```python
from build123d import *

# Parameters (mm, degrees)
F0_R     = 1
F1_DEPTH = 6.5


with BuildPart() as f1:
    # F0 (on Front) → F1 (new body)
    with BuildSketch(Plane.XZ):
        with BuildLine():
            ThreePointArc((-35.216109, -69.5), (-37.643365, -66.55518), (-40.997419, -68.375582))
            ThreePointArc((-40.997419, -68.375582), (-39.352976, -72.276245), (-35.444986, -70.649293))
            ThreePointArc((-35.444986, -70.649293), (-35.273885, -70.085931), (-35.216109, -69.5))
        make_face()
        with BuildLine():
            Line((4, 9.5), (-4, 9.5))
            Line((-4, 9.5), (-4, -6.441955))
            ThreePointArc((-4, -6.441955), (-4.516669, -9.27034), (-5.999941, -11.73339))
            ThreePointArc((-5.999941, -11.73339), (-25.901345, -38.569953), (-40.997419, -68.375582))
            ThreePointArc((-40.997419, -68.375582), (-37.643365, -66.55518), (-35.216109, -69.5))
            ThreePointArc((-35.216109, -69.5), (-35.273885, -70.085931), (-35.444986, -70.649293))
            ThreePointArc((-35.444986, -70.649293), (-18.875971, -40.819152), (4, -15.5))
            Line((4, -15.5), (4, -9.5))
            Line((4, -9.5), (4, 9.5))
        make_face()
        with Locations((0, -12.5)):
            Circle(F0_R, mode=Mode.SUBTRACT)
    extrude(amount=F1_DEPTH)


solid = f1.part
```
Check sheet for the modelled part. Datum: model origin and axes. Units: mm. Round coordinates to 2 decimals unless told otherwise and drop trailing zeros. Order: outer loops, then holes, each group sorted by start corner. A loop starts at its lowest first (then second) coordinate and runs counter-clockwise, first axis right, second up.
1) Section check C-C (z = -12.5). Record the boundary of the cut face in (x, y).
2) Scan lines: line 1 (X direction, y = -4, z = -1); line 2 (Z direction, x = 0, y = -3); line 3 (Z direction, x = -0.5, y = -3). Record each from-to range of solid material in increasing order.
3) Section check D-D (x = -37). Record the boundary of the cut face in (y, z), and give its area (3 significant figures).
4) Section check A-A (y = -5). Record the boundary of the cut face in (x, z), and give its area (3 significant figures).
5) Section check B-B (x = 0). Record the boundary of the cut face in (y, z), and give its area (3 significant figures).
6) Go/stop test with flat-tipped pins: pin 1 Ø3 at (y, z) = (-4, -49.5) entering from -X; pin 2 Ø1 at (y, z) = (-1, -54.5) entering from +X; pin 3 Ø1.5 at (x, y) = (-8.5, -2) entering from -Z. Record where each tip stops, or that it passes through.
7) Mould release check, pull along Z, two halves, no side actions. Record for faces 1 (the cylindrical face through (-19.154, -3.204, -41.209)), 2 (the flat face through (-4, -3, 2)), 3 (the cylindrical face through (0.46, -3.2, -13.39)): +Z half, -Z half, draft (parallel to the pull), parting line (faces both ways), or undercut.
Result:
1. outline: (-6.67, -6.5) - (-1, -6.5) - (-1, 0) - (-6.67, 0) - close; (1, -6.5) - (4, -6.5) - (4, 0) - (1, 0) - close
2. line 1: x = -4 to 4
2. line 2: z = -19.15 to -13.5, -11.5 to 9.5
2. line 3: z = -19.63 to -13.37, -11.63 to 9.5
3. outline: (-6.5, -72.24) - (0, -72.24) - (0, -59.17) - (-6.5, -59.17) - close
3. area: 85.0 mm2
4. outline: (-41, -68.38) arc R3 ccw to (-35.44, -70.65) arc R150.16 cw to (4, -15.5) - (4, 9.5) - (-4, 9.5) - (-4, -6.44) arc R8 cw to (-6, -11.73) arc R197.62 ccw to start; hole circle Ø2 at (0, -12.5)
4. area: 700 mm2
5. outline: (-6.5, -19.15) - (0, -19.15) - (0, -13.5) - (-6.5, -13.5) - close; (-6.5, -11.5) - (0, -11.5) - (0, 9.5) - (-6.5, 9.5) - close
5. area: 173 mm2
6. pin 1: stops at x = -32.97
6. pin 2: stops at x = -27.3
6. pin 3: stops at z = -28.73
7. face 1: -Z half
7. face 2: draft
7. face 3: undercut
